from build123d import *

# Parameters (mm, degrees)
STOCK_RECORD_NEEDLE_1_DEPTH     = 3.175
FILLET1_R                       = 3.175
X_Z_TURN_SKETCH_W               = 4.233333334
X_Z_TURN_SKETCH_H               = 3.81
X_Y_TURN_DEPTH                  = 3.175
FILLET2_R                       = 2.54
RIGHT_START                     = -3.175
RIGHT_SIDE_DELETE_DEPTH         = 3.175
SERVO_HORN_MOUNT_HOLES_SKETCH_R = 0.3175
SERVO_HORN_MOUNT_HOLES_DEPTH    = 157.399949281


# Read off the part's stored shape, not the designer's step: Stock-Record Needle-1
with BuildPart() as part:
    # Stock-Record Needle-1 outline → Stock-Record Needle-1 (new body)
    with BuildSketch(Plane(origin=(0, 0, 0), x_dir=(1, 0, 0), z_dir=(0, 1, 0))):
        with BuildLine():
            Line((-12.264516886, 3.297214818), (-88.464516886, 3.297214818))
            Line((-88.464516886, 3.297214818), (-122.158808708, 41.314772585))
            Line((-122.158808708, 41.314772585), (-122.158808708, 52.642883574))
            Line((-122.158808708, 52.642883574), (-134.794168142, 66.899467737))
            Line((-134.794168142, 66.899467737), (-141.955930631, 60.428744281))
            Line((-141.955930631, 60.428744281), (-141.955930631, 54.078744281))
            Line((-141.955930631, 54.078744281), (-91.321262361, -3.052785182))
            Line((-91.321262361, -3.052785182), (-12.327631672, -3.052785182))
            ThreePointArc((-12.327631672, -3.052785182), (12.699372727, -0.126223338), (-12.264516886, 3.297214818))
        make_face()
    extrude(amount=STOCK_RECORD_NEEDLE_1_DEPTH)

    # Fillet1
    fillet1_edges = [part.edges().sort_by_distance(p)[0] for p in [
        (-122.158808708, 1.5875, -52.642883574),
        (-134.794168142, 1.5875, -66.899467737),
        (-141.955930631, 1.5875, -60.428744281),
        (-141.955930631, 1.5875, -54.078744281),
        (-12.327631672, 1.5875, 3.052785182),
        (-12.264516886, 1.5875, -3.297214818),
        (-88.464516886, 1.5875, -3.297214818),
        (-122.158808708, 1.5875, -41.314772585),
        (-91.321262361, 1.5875, 3.052785182),
    ]]
    fillet(fillet1_edges, radius=FILLET1_R)

    # X-Z Turn Sketch' → X-Y Turn (add)
    with BuildSketch(Plane(origin=(0, 0, 0), x_dir=(1, 0, 0), z_dir=(0, 1, 0))):
        Polygon((-6.35, 34.29), (-2.116666667, 34.29), (-2.116666667, 38.1), (2.116666667, 38.1), (2.116666667, 34.29), (6.35, 34.29), (6.35, -34.29), (2.116666667, -34.29), (-2.116666667, -34.29), (-6.35, -34.29), align=None)
        with Locations((0, -36.195)):
            Rectangle(X_Z_TURN_SKETCH_W, X_Z_TURN_SKETCH_H)
    extrude(amount=X_Y_TURN_DEPTH)

    # Fillet2
    fillet2_edges = [part.edges().sort_by_distance(p)[0] for p in [
        (6.35, 1.5875, -10.998522627),
        (6.35, 1.5875, 10.998522628),
        (-6.35, 1.5875, -10.998522628),
        (-6.35, 1.5875, 10.998522629),
    ]]
    fillet(fillet2_edges, radius=FILLET2_R)

    # Sketch2 → Right Side Delete (cut)
    with BuildSketch(Plane(origin=(0, 3.175, 0), x_dir=(1, 0, 0), z_dir=(0, 1, 0)).offset(RIGHT_START)):
        with BuildLine():
            Line((11.695597813, 4.950049677), (11.695597813, 35.504326251))
            Line((11.695597813, 35.504326251), (11.695597813, 40.086272904))
            Line((11.695597813, 40.086272904), (-12.040083059, 40.086272904))
            Line((-12.040083059, 40.086272904), (-9.843545264, 8.024625639))
            ThreePointArc((-9.843545264, 8.024625639), (1.79465289, 12.572558252), (11.695597813, 4.950049677))
        make_face()
    extrude(amount=RIGHT_SIDE_DELETE_DEPTH, mode=Mode.SUBTRACT)

    # Servo Horn Mount Holes Sketch → Servo Horn Mount Holes (cut, through all)
    with BuildSketch(Plane.XZ):
        with Locations(Location((0, 8.1661, 0), (0, 0, 270))):
            Circle(SERVO_HORN_MOUNT_HOLES_SKETCH_R)
        with Locations(Location((2.794, 8.1661, 0), (0, 0, 270))):
            Circle(SERVO_HORN_MOUNT_HOLES_SKETCH_R)
        with Locations(Location((-2.794, 8.1661, 0), (0, 0, 270))):
            Circle(SERVO_HORN_MOUNT_HOLES_SKETCH_R)
        with Locations(Location((2.794, -8.279792428, 0), (0, 0, 90))):
            Circle(SERVO_HORN_MOUNT_HOLES_SKETCH_R)
        with Locations(Location((0, -8.279792428, 0), (0, 0, 90))):
            Circle(SERVO_HORN_MOUNT_HOLES_SKETCH_R)
        with Locations(Location((-2.794, -8.279792428, 0), (0, 0, 90))):
            Circle(SERVO_HORN_MOUNT_HOLES_SKETCH_R)
        with Locations(Location((8.1661, -0.113692428, 0), (0, 0, 270))):
            Circle(SERVO_HORN_MOUNT_HOLES_SKETCH_R)
        with Locations(Location((8.1661, 2.680307572, 0), (0, 0, 270))):
            Circle(SERVO_HORN_MOUNT_HOLES_SKETCH_R)
        with Locations(Location((8.1661, -2.907692428, 0), (0, 0, 270))):
            Circle(SERVO_HORN_MOUNT_HOLES_SKETCH_R)
        with Locations(Location((-8.1661, -2.907692428, 0), (0, 0, 90))):
            Circle(SERVO_HORN_MOUNT_HOLES_SKETCH_R)
        with Locations(Location((-8.1661, 2.680307572, 0), (0, 0, 90))):
            Circle(SERVO_HORN_MOUNT_HOLES_SKETCH_R)
        with Locations(Location((-8.1661, -0.113692428, 0), (0, 0, 90))):
            Circle(SERVO_HORN_MOUNT_HOLES_SKETCH_R)
    extrude(amount=-SERVO_HORN_MOUNT_HOLES_DEPTH, mode=Mode.SUBTRACT)


solid = part.part
Here's how the part is built. I have some questions about the finished solid (model axes, mm). A direction names the side the tool comes from. Round coordinates to 2 decimals unless told otherwise and drop trailing zeros. Write each loop counter-clockwise with the first axis right and the second up, starting at its lowest first coordinate (ties: lowest second). Pieces come first, ordered by that corner, then holes.
1. Will these pins go through, and if not, where does the flat tip stop? pin 1 Ø1.5 at (x, y) = (-73.5, 1) entering from -Z; pin 2 Ø1.6 at (x, y) = (-47, 1) entering from +Z; pin 3 Ø1 at (y, z) = (1, 36.5) entering from -X.
2. Suppose I cut it at C-C (z = -25). List the corners of the cut face in (x, y) for me (3 decimals), and give its area (3 significant figures).
3. I need wall thicknesses on L1, parallel to Z at x = -75, y = 2.75; L2, parallel to X at y = 2.9, z = 33; L3, parallel to X at y = 1.3, z = -41. Which ranges of each line are inside material? Lowest first, please.
4. For faces 1 (the flat face through (-53, 2, 3.053)), 2 (the flat face through (-105.162, 1.565, -22.138)), 3 (the flat face through (-122.159, 2, -47)), 4 (the flat face through (-139, 1.6, -63.1)), 5 (the flat face through (2.117, 2, 36)), which set-ups out of +Z, -Z, +X, -X, +Y, -Y let a thin tool reach every point of the face, with its end or its side?
5. Suppose I cut it at B-B (y = 0.5). State how many separate pieces and enclosed holes the cut face has, and give its area (3 significant figures).
6. Suppose I cut it at A-A (x = -38.5). List the corners of the cut face in (y, z) for me (3 decimals).
Answer sheet:
1. pin 1: stops at z = -3.3
1. pin 2: stops at z = 3.05
1. pin 3: stops at x = -2.12
2. outline: (-116.184, 0) - (-107.699, 0) - (-107.699, 3.175) - (-116.184, 3.175) - close
2. area: 26.9 mm2
3. L1: z = -3.3 to 3.05
3. L2: x = -6.35 to 6.35
3. L3: x = -130.36 to -121.77
4. face 1: +Z, -X, +Y, -Y
4. face 2: -Z, +Y, -Y
4. face 3: -Z, +X, +Y, -Y
4. face 4: -Z, -X, +Y, -Y
4. face 5: +Z, +X, +Y, -Y
5. separate pieces: 1
5. enclosed holes: 12
5. area: 1,960 mm2
6. outline: (0, -3.297) - (3.175, -3.297) - (3.175, 3.053) - (0, 3.053) - close
